For this review, use the dimensioned drawing (mm, ordinates from the lowest corner) and the shaded views. A direction names the side the tool comes from. Coordinates: 2 decimals unless noted, no trailing zeros. Order: outer loops, then holes, each group sorted by start corner. A loop starts at its lowest first (then second) coordinate and runs counter-clockwise, first axis right, second up. Notation, with made-up numbers: M 55,-33 L 95,-33 A8 ccw 95,-19 Z; hole C 70,73.25 d1. An arc over 180 degrees is marked long. Answer in a Markdown table with one row per item.
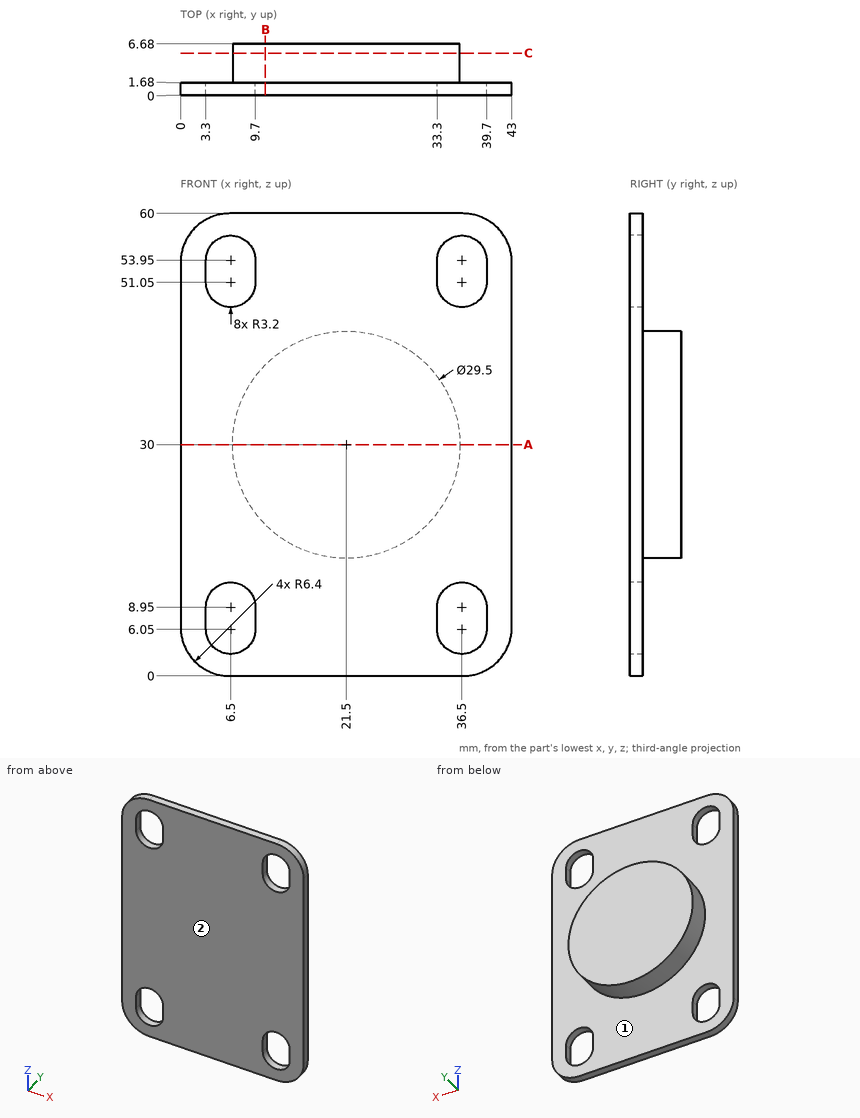
(1) To check wall thickness, follow line 1 (X direction, y = 1.5, z = 49); line 2 (Y direction, x = 28, z = 16); line 3 (Z direction, x = 38, y = 1) (3 decimals). State the ranges of each line that lie inside material, in increasing order. Write a range as [from, to].
Report:
| item | result |
|---|---|
| line 1 | [0, 4.04], [8.96, 34.04], [38.96, 43] |
| line 2 | [0, 1.68] |
| line 3 | [0.155, 3.223], [11.777, 48.223], [56.777, 59.845] |
(2) Take a section at C-C (y = 5.5). Write out the cut boundary in (x, z), then the cut area to 3 significant figures.
Report:
| item | result |
|---|---|
| outline | C 21.5,30 d29.5 |
| area | 683 mm^2 |
(3) Take a section at A-A (z = 30). Write out the cut boundary in (x, y).
Report:
| item | result |
|---|---|
| outline | M 0,0 L 43,0 L 43,1.68 L 36.25,1.68 L 36.25,6.68 L 6.75,6.68 L 6.75,1.68 L 0,1.68 Z |
(4) Machinability: for the marked faces 1 and 2, which of the approach directions +Z, -Z, +X, -X, +Y, -Y give a long, thin tool a straight path to every point of the face, cutting with its end or side? Answer none if there is none.
Report:
| item | result |
|---|---|
| face 1 | +Y |
| face 2 | +Z, -Z, +X, -X, -Y |
(5) Take a section at B-B (x = 11). Write out the cut boundary in (y, z), then the cut area to 3 significant figures.
Report:
| item | result |
|---|---|
| outline | M 0,0 L 1.68,0 L 1.68,19.64 L 6.68,19.64 L 6.68,40.36 L 1.68,40.36 L 1.68,60 L 0,60 Z |
| area | 204 mm^2 |
